```python
from build123d import *

# Parameters (mm, degrees)
SKETCH1_R           = 32.766
BOSS_EXTRUDE1_DEPTH = 38.1


with BuildPart() as part:
    # Sketch1 → Boss-Extrude1 (new body)
    with BuildSketch(Plane.XY):
        with BuildLine():
            ThreePointArc((45.466, 134.62), (0, 180.086), (-45.466, 134.62))
            Line((-45.466, 134.62), (-45.466, -36.83))
            Line((-45.466, -36.83), (45.472760733, -36.83))
            Line((45.472760733, -36.83), (45.472760733, 0))
            Line((45.472760733, 0), (45.466, 134.62))
        make_face()
        with Locations(Location((0, 0, 0), (0, 0, 180))):
            Circle(SKETCH1_R, mode=Mode.SUBTRACT)
        with BuildLine():
            Line((-40.386, 20.883681668), (-40.386, 46.426318332))
            ThreePointArc((-40.386, 46.426318332), (-38.829045243, 43.657042436), (-37.082505751, 41.003253275))
            ThreePointArc((-37.082505751, 41.003253275), (-34.740747581, 33.655), (-37.082505751, 26.306746725))
            ThreePointArc((-37.082505751, 26.306746725), (-38.829045243, 23.652957564), (-40.386, 20.883681668))
        make_face(mode=Mode.SUBTRACT)
        with Locations(Location((0, 67.31, 0), (0, 0, 180))):
            Circle(SKETCH1_R, mode=Mode.SUBTRACT)
        with BuildLine():
            ThreePointArc((37.082505751, 41.003253275), (38.831553537, 43.661160581), (40.390428727, 46.434885072))
            Line((40.390428727, 46.434885072), (40.391709837, 20.925359586))
            ThreePointArc((40.391709837, 20.925359586), (39.020141495, 23.38352957), (37.499160948, 25.752161572))
            ThreePointArc((37.499160948, 25.752161572), (34.745484352, 33.308169261), (37.082505751, 41.003253275))
        make_face(mode=Mode.SUBTRACT)
        with BuildLine():
            Line((-40.386, 88.193681668), (-40.386, 113.736318332))
            ThreePointArc((-40.386, 113.736318332), (-38.829045243, 110.967042436), (-37.082505751, 108.313253275))
            ThreePointArc((-37.082505751, 108.313253275), (-34.740747581, 100.965), (-37.082505751, 93.616746725))
            ThreePointArc((-37.082505751, 93.616746725), (-38.829045243, 90.962957564), (-40.386, 88.193681668))
        make_face(mode=Mode.SUBTRACT)
        with Locations(Location((0, 134.62, 0), (0, 0, 180))):
            Circle(SKETCH1_R, mode=Mode.SUBTRACT)
        with BuildLine():
            ThreePointArc((37.082505751, 108.313253275), (38.829639134, 110.968017404), (40.387048688, 113.738346468))
            Line((40.387048688, 113.738346468), (40.38833179, 88.189171708))
            ThreePointArc((40.38833179, 88.189171708), (38.830365823, 90.960789544), (37.082505751, 93.616746725))
            ThreePointArc((37.082505751, 93.616746725), (34.740747581, 100.965), (37.082505751, 108.313253275))
        make_face(mode=Mode.SUBTRACT)
    extrude(amount=BOSS_EXTRUDE1_DEPTH)


solid = part.part
```
Build history of the part. All positions in model axes, mm. A direction names the side the tool comes from. Give positions to 0.01 mm unless a question says otherwise; leave off trailing zeros. Loops run counter-clockwise (first coordinate to the right, second up) from the corner with the lowest first, then second, coordinate; pieces in that order, holes last.
Item 1: Drill centre lines: line 1 (Y direction, x = 0, z = 10.5); line 2 (X direction, y = 134.62, z = 15.5); line 3 (Y direction, x = -24.5, z = 35.5). Where is each one in solid material? Low to high.
Answers follow:
line 1: y = -36.83 to -32.77, 32.77 to 34.54, 100.08 to 101.85, 167.39 to 180.09
line 2: x = -45.47 to -32.77, 32.77 to 45.47
line 3: y = -36.83 to -21.76, 21.76 to 45.55, 89.07 to 112.86, 156.38 to 172.92
Item 2: Slice it at C-C, the plane y = 123. List the corners of the cut face in (x, z).
Answers follow:
outline: (-45.47, 0) - (-30.64, 0) - (-30.64, 38.1) - (-45.47, 38.1) - close; (30.64, 0) - (45.47, 0) - (45.47, 38.1) - (30.64, 38.1) - close
Item 3: Pull direction Y, two halves, no side cores. Call faces 3 (the face through (-1, -36.83, 19)), 4 (the face through (-38.8, 23.7, 18.8)), 5 (the face through (7.103, 166.607, 18.783)), 6 (the face through (1, 180.075, 18.783)): released by +Y, released by -Y, zero draft, split by the parting line, or undercut.
Answers follow:
face 3: released by -Y
face 4: undercut
face 5: undercut
face 6: released by +Y
Item 4: Slice it at B-B, the plane z = 15. List the corners of the cut face in (x, y) (1 decimal), and give its area (3 significant figures).
Answers follow:
outline: (-45.5, -36.8) - (45.5, -36.8) - (45.5, 0) - (45.5, 134.6) arc R45.5 ccw to (-45.5, 134.6) - close; hole (-40.4, 20.9) arc R45.5 cw to (-37.1, 26.3) arc R12.7 ccw to (-37.1, 41) arc R45.5 cw to (-40.4, 46.4) - close; hole (-40.4, 88.2) arc R45.5 cw to (-37.1, 93.6) arc R12.7 ccw to (-37.1, 108.3) arc R45.5 cw to (-40.4, 113.7) - close; hole circle Ø65.5 at (0, 0); hole circle Ø65.5 at (0, 67.3); hole circle Ø65.5 at (0, 134.6); hole (37.1, 41) arc R12.7 ccw to (37.5, 25.8) arc R45.5 cw to (40.4, 20.9) - (40.4, 46.4) arc R45.5 cw to start; hole (37.1, 93.6) arc R45.5 cw to (40.4, 88.2) - (40.4, 113.7) arc R45.5 cw to (37.1, 108.3) arc R12.7 ccw to start
area: 8,360 mm2
Item 5: Which spindle directions (+Z, -Z, +X, -X, +Y, -Y) get a long thin tool onto all of the face, cutting with end or side? Do faces 1 (the face through (-21, 97, 38.1)), 2 (the face through (-34.74, 33.76, 18.78)). Say none if no direction does.
Answers follow:
face 1: +Z, +X, -X, +Y, -Y
face 2: +Z, -Z
Item 6: Flat gauge pins, fed straight in: pin 1 (4 mm diameter, centred on x = 30.5, z = 10.5, fed in from +Y); pin 2 (10 mm diameter, centred on x = 34, z = 10, fed in from +Y); pin 3 (2 mm diameter, centred on x = 11.5, z = 28.5, fed in from +Y). Where does each tip first touch, or does it go through?
Answers follow:
pin 1: stops at y = 170.04
pin 2: stops at y = 169.64
pin 3: stops at y = 178.86
Item 7: Slice it at D-D, the plane y = 152. List the corners of the cut face in (x, z).
Answers follow:
outline: (-42.01, 0) - (-27.78, 0) - (-27.78, 38.1) - (-42.01, 38.1) - close; (27.78, 0) - (42.01, 0) - (42.01, 38.1) - (27.78, 38.1) - close
Item 8: Slice it at A-A, the plane x = 0. List the corners of the cut face in (y, z), and give its area (3 significant figures).
Answers follow:
outline: (-36.83, 0) - (-32.77, 0) - (-32.77, 38.1) - (-36.83, 38.1) - close; (32.77, 0) - (34.54, 0) - (34.54, 38.1) - (32.77, 38.1) - close; (100.08, 0) - (101.85, 0) - (101.85, 38.1) - (100.08, 38.1) - close; (167.39, 0) - (180.09, 0) - (180.09, 38.1) - (167.39, 38.1) - close
area: 774 mm2
